from build123d import *

# Parameters (mm, degrees)
SKETCH_1_W          = 99.656546146
SKETCH_1_H          = 91.603491912
SKETCH_1_W_2        = 60.1
SKETCH_1_H_2        = 75.5
EXTRUDE_1_DEPTH     = 5
SKETCH_2_R          = 1.55
CUT_EXTRUDE_1_DEPTH = 5
SKETCH_3_R          = 1.5
CUT_EXTRUDE_2_DEPTH = 5


with BuildPart() as part:
    # 草图1 → 凸台-拉伸1 (new body)
    with BuildSketch(Plane(origin=(0, 0, 0), x_dir=(1, 0, 0), z_dir=(0, 1, 0))):
        with Locations((1.039363494, -3.201523692)):
            Rectangle(SKETCH_1_W, SKETCH_1_H)
        Rectangle(SKETCH_1_W_2, SKETCH_1_H_2, mode=Mode.SUBTRACT)
    extrude(amount=EXTRUDE_1_DEPTH)

    # 草图2 → 切除-拉伸1 (cut)
    with BuildSketch(Plane(origin=(0, 5, 0), x_dir=(1, 0, 0), z_dir=(0, 1, 0))):
        with Locations(Location((35, 30.369317712, 0), (0, 0, 270))):
            Circle(SKETCH_2_R)
        with Locations(Location((35, -30.369317712, 0), (0, 0, 270))):
            Circle(SKETCH_2_R)
        with Locations(Location((-35, -30.369317712, 0), (0, 0, 270))):
            Circle(SKETCH_2_R)
        with Locations(Location((-35, 30.369317712, 0), (0, 0, 270))):
            Circle(SKETCH_2_R)
    extrude(amount=-CUT_EXTRUDE_1_DEPTH, mode=Mode.SUBTRACT)

    # 草图3 → 切除-拉伸2 (cut)
    with BuildSketch(Plane(origin=(0, 5, 0), x_dir=(1, 0, 0), z_dir=(0, 1, 0))):
        with Locations((28.55, -37.75)):
            Circle(SKETCH_3_R)
        with Locations((28.55, 37.75)):
            Circle(SKETCH_3_R)
        with Locations((-28.55, 37.75)):
            Circle(SKETCH_3_R)
        with Locations((-28.55, -37.75)):
            Circle(SKETCH_3_R)
    extrude(amount=-CUT_EXTRUDE_2_DEPTH, mode=Mode.SUBTRACT)


solid = part.part
Input: part model. Units: mm. Frame: model coordinates. A direction names the side the tool comes from. Give positions to 0.01 mm unless a question says otherwise; leave off trailing zeros. Write each loop counter-clockwise with the first axis right and the second up, starting at its lowest first coordinate (ties: lowest second). Pieces come first, ordered by that corner, then holes.
Q1. Section B-B, the plane z = 2. Output: boundary loops of the cut face in (x, y), plus the area to 3 significant figures.
Q2. Set-up query: faces 4 (the face through (0, 2, -42.6)), 5 (the face through (-28.52, 2.54, -39.25)). Return all of +Z, -Z, +X, -X, +Y, -Y with unobstructed straight access to the full face (end or side cutting, diameter ignored); none if empty.
Q3. Section A-A, the plane x = -11.5. Output: boundary loops of the cut face in (y, z), plus the area to 3 significant figures.
Q4. Material intervals for probe 1 along X at (y, z) = (4.45, 16.5); probe 2 along Z at (x, y) = (-25, 3.4); probe 3 along Z at (x, y) = (-29, 3.8), sorted ascending.
Q5. Pull-direction query (X, two-part tool) for faces 1 (the face through (-33, 5, 3)), 2 (the face through (50.868, 2, 4)), 3 (the face through (-30.05, 2, 1)); classes: pulls with the +X half, pulls with the -X half, needs draft (parallel to the pull), parting line crosses it, or undercut.
Q6. First-contact query: P1, Ø3.5, axis at x = 35, z = 30.37, coming from the -Y side. Flat tip, straight axial feed; report the tip coordinate or a pass-through.
Q7. Section D-D, the plane x = 35. Output: boundary loops of the cut face in (y, z).
Q8. Section C-C, the plane y = 2.35. Output: boundary loops of the cut face in (x, z).
Filled in:
1. outline: (-48.79, 0) - (-30.05, 0) - (-30.05, 5) - (-48.79, 5) - close; (30.05, 0) - (50.87, 0) - (50.87, 5) - (30.05, 5) - close
1. area: 198 mm2
2. face 4: -Z, +X, -X, +Y, -Y
2. face 5: +Y, -Y
3. outline: (0, -42.6) - (5, -42.6) - (5, -37.75) - (0, -37.75) - close; (0, 37.75) - (5, 37.75) - (5, 49) - (0, 49) - close
3. area: 80.5 mm2
4. probe 1: x = -48.79 to -30.05, 30.05 to 50.87
4. probe 2: z = -42.6 to -37.75, 37.75 to 49
4. probe 3: z = -42.6 to -39.18, 39.18 to 49
5. face 1: needs draft
5. face 2: pulls with the +X half
5. face 3: undercut
6. P1: stops at y = 0
7. outline: (0, -42.6) - (5, -42.6) - (5, -31.92) - (0, -31.92) - close; (0, -28.82) - (5, -28.82) - (5, 28.82) - (0, 28.82) - close; (0, 31.92) - (5, 31.92) - (5, 49) - (0, 49) - close
8. outline: (-48.79, -42.6) - (50.87, -42.6) - (50.87, 49) - (-48.79, 49) - close; hole circle Ø3.1 at (-35, -30.37); hole circle Ø3.1 at (-35, 30.37); hole (-30.05, -37.75) arc R1.5 ccw to (-27.05, -37.75) - (27.05, -37.75) arc R1.5 ccw to (30.05, -37.75) - (30.05, 37.75) arc R1.5 ccw to (27.05, 37.75) - (-27.05, 37.75) arc R1.5 ccw to (-30.05, 37.75) - close; hole circle Ø3.1 at (35, -30.37); hole circle Ø3.1 at (35, 30.37)
